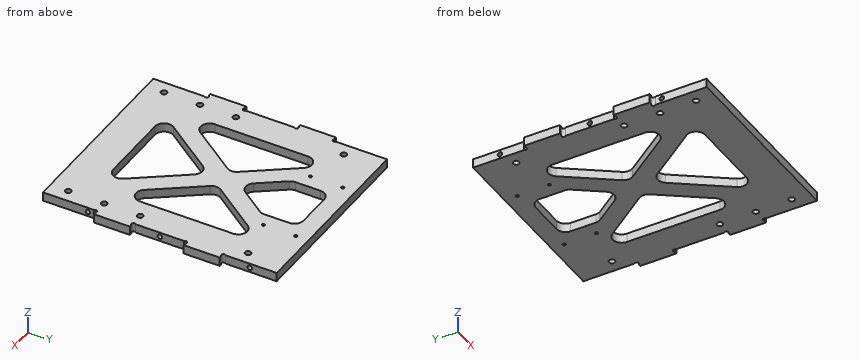
from build123d import *

# Parameters (mm, degrees)
EXTRUDE_1_DEPTH     = 5
SKETCH_2_R          = 1.25
CUT_EXTRUDE_1_DEPTH = 10
SKETCH_3_R          = 1.65
CUT_EXTRUDE_2_DEPTH = 10
SKETCH_5_R          = 0.8
CUT_EXTRUDE_4_DEPTH = 10
CUT_EXTRUDE_3_DEPTH = 10
FILLET_2_R          = 5


with BuildPart() as part:
    # ｽｹｯﾁ1 → ﾎﾞｽ - 押し出し1 (new body)
    with BuildSketch(Plane.XY):
        with BuildLine():
            Line((-53, -40.640312424), (-53, -65))
            Line((-53, -65), (53, -65))
            Line((53, -65), (53, -40.640312424))
            ThreePointArc((53, -40.640312424), (52.9, -40), (53, -39.359687576))
            Line((53, -39.359687576), (53, -36.54))
            ThreePointArc((53, -36.54), (52.882182541, -34.882182541), (54.54, -35))
            Line((54.54, -35), (56, -35))
            Line((56, -35), (56, -15))
            Line((56, -15), (54.54, -15))
            ThreePointArc((54.54, -15), (52.882182541, -15.117817459), (53, -13.46))
            Line((53, -13.46), (53, -0.640312424))
            ThreePointArc((53, -0.640312424), (52.9, 0), (53, 0.640312424))
            Line((53, 0.640312424), (53, 13.46))
            ThreePointArc((53, 13.46), (52.882182541, 15.117817459), (54.54, 15))
            Line((54.54, 15), (56, 15))
            Line((56, 15), (56, 35))
            Line((56, 35), (54.54, 35))
            ThreePointArc((54.54, 35), (52.882182541, 34.882182541), (53, 36.54))
            Line((53, 36.54), (53, 49.359687576))
            ThreePointArc((53, 49.359687576), (52.9, 50), (53, 50.640312424))
            Line((53, 50.640312424), (53, 65))
            Line((53, 65), (-53, 65))
            Line((-53, 65), (-53, 50.640312424))
            ThreePointArc((-53, 50.640312424), (-52.9, 50), (-53, 49.359687576))
            Line((-53, 49.359687576), (-53, 36.54))
            ThreePointArc((-53, 36.54), (-52.882182541, 34.882182541), (-54.54, 35))
            Line((-54.54, 35), (-56, 35))
            Line((-56, 35), (-56, 15))
            Line((-56, 15), (-54.54, 15))
            ThreePointArc((-54.54, 15), (-52.882182541, 15.117817459), (-53, 13.46))
            Line((-53, 13.46), (-53, 0.640312424))
            ThreePointArc((-53, 0.640312424), (-52.9, 0), (-53, -0.640312424))
            Line((-53, -0.640312424), (-53, -13.46))
            ThreePointArc((-53, -13.46), (-52.882182541, -15.117817459), (-54.54, -15))
            Line((-54.54, -15), (-56, -15))
            Line((-56, -15), (-56, -35))
            Line((-56, -35), (-54.54, -35))
            ThreePointArc((-54.54, -35), (-52.882182541, -34.882182541), (-53, -36.54))
            Line((-53, -36.54), (-53, -39.359687576))
            ThreePointArc((-53, -39.359687576), (-52.9, -40), (-53, -40.640312424))
        make_face()
    extrude(amount=EXTRUDE_1_DEPTH)

    # ｽｹｯﾁ2 → ｶｯﾄ - 押し出し1 (cut)
    with BuildSketch(Plane.ZY.offset(53)):
        with Locations((2.5, -40)):
            Circle(SKETCH_2_R)
        with Locations((2.5, 0)):
            Circle(SKETCH_2_R)
        with Locations((2.5, 50)):
            Circle(SKETCH_2_R)
    cut_extrude_1 = extrude(amount=-CUT_EXTRUDE_1_DEPTH, mode=Mode.SUBTRACT)

    # ﾐﾗｰ1: ｶｯﾄ - 押し出し1 across plane
    add(cut_extrude_1.mirror(Plane(origin=(0, 0, 0), x_dir=(0, 0, 1), z_dir=(1, 0, 0))), mode=Mode.SUBTRACT)

    # ｽｹｯﾁ3 → ｶｯﾄ - 押し出し2 (cut)
    with BuildSketch(Plane.XY.offset(5)):
        with Locations((-46, -55)):
            Circle(SKETCH_3_R)
        with Locations((46, -55)):
            Circle(SKETCH_3_R)
        with Locations((46, -35)):
            Circle(SKETCH_3_R)
        with Locations((-46, -35)):
            Circle(SKETCH_3_R)
        with Locations((-46, -15)):
            Circle(SKETCH_3_R)
        with Locations((46, -15)):
            Circle(SKETCH_3_R)
        with Locations((-46, 45)):
            Circle(SKETCH_3_R)
        with Locations((46, 45)):
            Circle(SKETCH_3_R)
    extrude(amount=-CUT_EXTRUDE_2_DEPTH, mode=Mode.SUBTRACT)

    # ｽｹｯﾁ5 → ｶｯﾄ - 押し出し4 (cut)
    with BuildSketch(Plane.XY.offset(5)):
        with Locations((-22.6, 40)):
            Circle(SKETCH_5_R)
        with Locations((22.6, 40)):
            Circle(SKETCH_5_R)
        with Locations((22.6, 58)):
            Circle(SKETCH_5_R)
        with Locations((-22.6, 58)):
            Circle(SKETCH_5_R)
    extrude(amount=-CUT_EXTRUDE_4_DEPTH, mode=Mode.SUBTRACT)

    # ｽｹｯﾁ4 → ｶｯﾄ - 押し出し3 (cut)
    with BuildSketch(Plane.XY.offset(5)):
        Polygon((-36, -36.442821222), (-6.16116872, 5), (-36, 46.442821222), align=None)
        Polygon((36, 46.442821222), (6.16116872, 5), (36, -36.442821222), align=None)
        Polygon((29.83883128, -45), (0, -3.557178778), (-29.83883128, -45), align=None)
        Polygon((15, 55), (-15, 55), (-15, 34.390512112), (0, 13.557178778), (15, 34.390512112), align=None)
    extrude(amount=-CUT_EXTRUDE_3_DEPTH, mode=Mode.SUBTRACT)

    # ﾌｨﾚｯﾄ2
    fillet_2_edges = [part.edges().sort_by_distance(p)[0] for p in [
        (-29.83883128, -45, 2.5),
        (0, -3.557178778, 2.5),
        (29.83883128, -45, 2.5),
        (6.16116872, 5, 2.5),
        (36, 46.442821222, 2.5),
        (36, -36.442821222, 2.5),
        (15, 55, 2.5),
        (15, 34.390512112, 2.5),
        (0, 13.557178778, 2.5),
        (-15, 34.390512112, 2.5),
        (-15, 55, 2.5),
        (-36, -36.442821222, 2.5),
        (-36, 46.442821222, 2.5),
        (-6.16116872, 5, 2.5),
    ]]
    fillet(fillet_2_edges, radius=FILLET_2_R)


solid = part.part
Input: part model. Units: mm. Frame: model coordinates. Give positions to 0.01 mm unless a question says otherwise; leave off trailing zeros. Order: outer loops, then holes, each group sorted by start corner. A loop starts at its lowest first (then second) coordinate and runs counter-clockwise, first axis right, second up. Notation, with made-up numbers: (4.25, 40.25) - (44.25, 40.25) arc R31 cw to (44.25, 73.25) - close; hole circle Ø7 at (-18.5, -3). An arc over 180 degrees is marked (long way). Answer as a JSON object with one key per item and string values. Group by question number.
Q1. Cut plane A-A, the plane x = 46. Output: boundary loops of the cut face in (y, z), then the cut area to 3 significant figures.
Q2. Cut plane D-D, the plane x = 1. Output: boundary loops of the cut face in (y, z).
Q3. Cut plane C-C, the plane x = -34.5. Output: boundary loops of the cut face in (y, z).
Q4. First-contact query: pin 1 Ø1.4 at (y, z) = (-38.5, 2.5) entering from +X; pin 2 Ø1.5 at (y, z) = (44.5, 1.5) entering from -X; pin 3 Ø2 at (y, z) = (0, 2.5) entering from -X. Flat tips, straight axial feed; report the tip coordinate or a pass-through.
Q5. Line query: probe 1 along X at (y, z) = (-6, 4.2); probe 2 along X at (y, z) = (40, 0.8); probe 3 along Y at (x, z) = (-53.66, 1.35). Output: solid intervals per line, ascending.
Q6. Cut plane B-B, the plane y = 45. Output: boundary loops of the cut face in (x, z).
Results:
{
 "1": {"outline": "(-65, 0) - (-56.65, 0) - (-56.65, 5) - (-65, 5) - close; (-53.35, 0) - (-36.65, 0) - (-36.65, 5) - (-53.35, 5) - close; (-33.35, 0) - (-16.65, 0) - (-16.65, 5) - (-33.35, 5) - close; (-13.35, 0) - (43.35, 0) - (43.35, 5) - (-13.35, 5) - close; (46.65, 0) - (65, 0) - (65, 5) - (46.65, 5) - close; hole circle Ø2.5 at (-40, 2.5); hole circle Ø2.5 at (0, 2.5); hole circle Ø2.5 at (50, 2.5)", "area": "569 mm^2"},
 "2": {"outline": "(-65, 0) - (-45, 0) - (-45, 5) - (-65, 5) - close; (-7.22, 0) - (17.22, 0) - (17.22, 5) - (-7.22, 5) - close; (55, 0) - (65, 0) - (65, 5) - (55, 5) - close"},
 "3": {"outline": "(-65, 0) - (-24.51, 0) - (-24.51, 5) - (-65, 5) - close; (34.51, 0) - (65, 0) - (65, 5) - (34.51, 5) - close"},
 "4": {"pin 1": "x = 53", "pin 2": "x = -53", "pin 3": "x = -43"},
 "5": {"probe 1": "-53 to -36, -14.08 to 14.08, 36 to 53", "probe 2": "-53 to -23.4, -21.8 to -15, 15 to 21.8, 23.4 to 53", "probe 3": "-34.56 to -15.44, 15.44 to 34.56"},
 "6": {"outline": "(-53, 0) - (-47.65, 0) - (-47.65, 5) - (-53, 5) - close; (-44.35, 0) - (-15, 0) - (-15, 5) - (-44.35, 5) - close; (15, 0) - (44.35, 0) - (44.35, 5) - (15, 5) - close; (47.65, 0) - (53, 0) - (53, 5) - (47.65, 5) - close"}
}
